Can you work these out from the model? Positions are in its coordinate system, mm. Face numbers are marked on the shaded views. A direction names the side the tool comes from. Coordinates: 2 decimals unless noted, no trailing zeros. Order: outer loops, then holes, each group sorted by start corner. A loop starts at its lowest first (then second) coordinate and runs counter-clockwise, first axis right, second up. Notation, with made-up numbers: (52.5, 48) -> (62.5, 48) arc R22 cw to (62.5, 74) -> close; hole circle Ø1 at (43.5, 33.5). An arc over 180 degrees is marked (long way). Use a Markdown table: item, result. Add a question column.
1. Suppose I cut it at D-D, the plane x = 20.5. List the corners of the cut face in (y, z) for me.
2. For pin 1 Ø1.5 at (y, z) = (2.5, -11) entering from +X; pin 2 Ø6 at (y, z) = (10, -26) entering from -X (3 decimals); pin 3 Ø4 at (x, y) = (-3, 5) entering from -Z, each with a flat end and sliding along its axis, tell me the tip position at first contact or that it passes through.
3. Suppose I cut it at C-C, the plane z = -9.75. List the corners of the cut face in (x, y) for me.
4. Suppose I cut it at A-A, the plane x = -2.4. List the corners of the cut face in (y, z) for me.
5. Suppose I cut it at B-B, the plane y = 10. List the corners of the cut face in (x, z) for me.
6. For the marked faces 1, 2 and 3, which set-ups out of +Z, -Z, +X, -X, +Y, -Y let a thin tool reach every point of the face, with its end or its side?
7. If I drill on line 1 along Y through (x, z) = (-2.4, -16.8); line 2 along Z through (x, y) = (14.5, 4.75); line 3 along X through (y, z) = (5.9, -16.4), over which ranges is the centre line in solid material (lowest first)? Write a range as from..to.
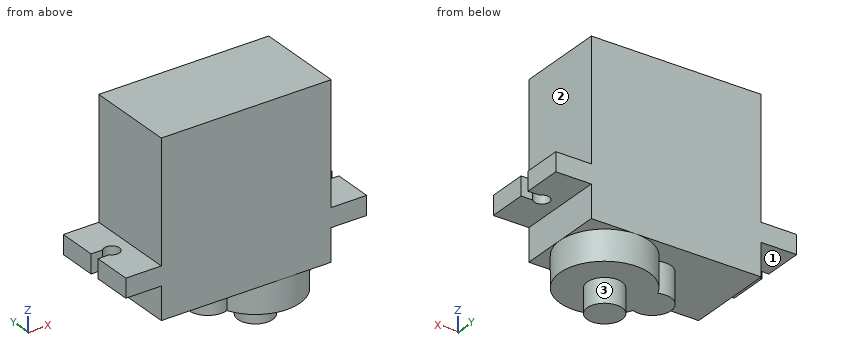
```python
from build123d import *

# Parameters (mm, degrees)
SKETCH1_W           = 22.5
SKETCH1_H           = 22.7
BOSS_EXTRUDE1_DEPTH = 11.8
SKETCH2_W           = 31.9
SKETCH2_H           = 2.5
BOSS_EXTRUDE2_DEPTH = 11.8
BOSS_EXTRUDE3_DEPTH = 4
SKETCH4_R           = 2.3
BOSS_EXTRUDE4_DEPTH = 3.2
CUT_EXTRUDE1_DEPTH  = 3.2


with BuildPart() as part:
    # Sketch1 → Boss-Extrude1 (new body)
    with BuildSketch(Plane(origin=(0, 0, 0), x_dir=(1, 0, 0), z_dir=(0, 1, 0))):
        with Locations((11.25, 11.35)):
            Rectangle(SKETCH1_W, SKETCH1_H)
    extrude(amount=BOSS_EXTRUDE1_DEPTH)

    # Sketch2 → Boss-Extrude2 (add)
    with BuildSketch(Plane(origin=(0, 11.8, 0), x_dir=(1, 0, 0), z_dir=(0, 1, 0))):
        with Locations((11.25, 17.15)):
            Rectangle(SKETCH2_W, SKETCH2_H)
    extrude(amount=-BOSS_EXTRUDE2_DEPTH)

    # Sketch3 → Boss-Extrude3 (add)
    with BuildSketch(Plane(origin=(0, 0, -22.7), x_dir=(-1, 0, 0), z_dir=(0, 0, -1))):
        with BuildLine():
            ThreePointArc((-11.183333333, 8.238743727), (-22.5, 5.9), (-11.183333333, 3.561256273))
            ThreePointArc((-11.183333333, 3.561256273), (-7.8, 5.9), (-11.183333333, 8.238743727))
        make_face()
    extrude(amount=BOSS_EXTRUDE3_DEPTH)

    # Sketch4 → Boss-Extrude4 (add)
    with BuildSketch(Plane(origin=(0, 0, -26.7), x_dir=(-1, 0, 0), z_dir=(0, 0, -1))):
        with Locations((-16.6, 5.9)):
            Circle(SKETCH4_R)
    extrude(amount=BOSS_EXTRUDE4_DEPTH)

    # Sketch5 → Cut-Extrude1 (cut)
    with BuildSketch(Plane(origin=(0, 0, -18.4), x_dir=(-1, 0, 0), z_dir=(0, 0, -1))):
        with BuildLine():
            Line((-27.2, 5.25), (-27.2, 6.55))
            Line((-27.2, 6.55), (-25.659934208, 6.55))
            ThreePointArc((-25.659934208, 6.55), (-23.9, 5.9), (-25.659934208, 5.25))
            Line((-25.659934208, 5.25), (-27.2, 5.25))
        make_face()
        with BuildLine():
            Line((4.7, 5.25), (3.159934208, 5.25))
            ThreePointArc((3.159934208, 5.25), (1.4, 5.9), (3.159934208, 6.55))
            Line((3.159934208, 6.55), (4.7, 6.55))
            Line((4.7, 6.55), (4.7, 5.25))
        make_face()
    extrude(amount=-CUT_EXTRUDE1_DEPTH, mode=Mode.SUBTRACT)


solid = part.part
```
Worked out:
| question | item | result |
|---|---|---|
| 1 | outline | (0, -22.7) -> (1.47, -22.7) -> (1.47, -26.7) -> (10.33, -26.7) -> (10.33, -22.7) -> (11.8, -22.7) -> (11.8, 0) -> (0, 0) -> close |
| 2 | pin 1 | stops at x = 22.5 |
| 2 | pin 2 | stops at x = 8.055 |
| 2 | pin 3 | stops at z = -18.4 |
| 3 | outline | (0, 0) -> (22.5, 0) -> (22.5, 11.8) -> (0, 11.8) -> close |
| 4 | outline | (0, -18.4) -> (4.9, -18.4) -> (4.9, -15.9) -> (0, -15.9) -> close; (6.9, -18.4) -> (11.8, -18.4) -> (11.8, -15.9) -> (6.9, -15.9) -> close |
| 5 | outline | (-4.7, -18.4) -> (0, -18.4) -> (0, -22.7) -> (12.36, -22.7) -> (12.36, -26.7) -> (20.84, -26.7) -> (20.84, -22.7) -> (22.5, -22.7) -> (22.5, -18.4) -> (27.2, -18.4) -> (27.2, -15.9) -> (22.5, -15.9) -> (22.5, 0) -> (0, 0) -> (0, -15.9) -> (-4.7, -15.9) -> close |
| 6 | face 1 | -Z, -X, +Y, -Y |
| 6 | face 2 | +Z, +X, +Y, -Y |
| 6 | face 3 | -Z |
| 7 | line 1 | y = 0..4.9, 6.9..11.8 |
| 7 | line 2 | z = -26.7..0 |
| 7 | line 3 | x = -1.4..23.9 |
